The model under review builds one solid part; all positions refer to its coordinate system, in mm. A direction names the side the tool comes from. Coordinates: 2 decimals unless noted, no trailing zeros. Write each loop counter-clockwise with the first axis right and the second up, starting at its lowest first coordinate (ties: lowest second). Pieces come first, ordered by that corner, then holes. Notation, with made-up numbers: (-35, -29) - (-30, -29) arc R16 cw to (-30, -6) - close; hole circle Ø11 at (76, -34.75). An arc over 180 degrees is marked (long way). Put each result on its own line as item: value. Start each with the question number.
Item 1: Mouldability with a two-part tool opening along Y and no side actions: class faces 1 (the face through (-4.5, 0, 2)), 2 (the face through (0, -2.25, 2)), 3 (the face through (2, -1.75, 2)) as pulls with the +Y half, pulls with the -Y half, needs draft (parallel to the pull), parting line crosses it, or undercut.
Item 2: Consider section C-C on z = 4.3. State how many separate pieces and enclosed holes the cut face has, then the cut area to 3 significant figures.
Item 3: For pin 1 (1.8 mm diameter, centred on x = 2, y = -0.5, fed in from +Z), flat-tipped, find the tip position at first contact; note if it passes through.
Item 4: Consider section B-B on y = 1.6. Give the boundary of the cut face in (x, z), then the cut area to 3 significant figures.
Item 5: Machinability: for faces 4 (the face through (0, 0, -0.5)), 5 (the face through (-4, 0, 2)), which of the approach directions +Z, -Z, +X, -X, +Y, -Y give a long, thin tool a straight path to every point of the face, cutting with its end or side? Answer none if there is none.
Item 6: To check wall thickness, follow L1, parallel to X at y = -1.5, z = 3.6; L2, parallel to Y at x = -2.25, z = 3.5; L3, parallel to Y at x = 1.75, z = 4.5. State the ranges of each line that lie inside material, in increasing order. Write a range as [from, to].
Item 7: Consider section A-A on z = 1.6. Give the boundary of the cut face in (x, y).
```python
from build123d import *

# Parameters (mm, degrees)
SKETCH1_W             = 0.5
SKETCH1_H             = 4.5
EXTRUDE_THIN2_DEPTH   = 5
SKETCH1_W_2           = 9
SKETCH1_W_3           = 8
SKETCH1_H_2           = 3.5
EXTRUDE_THIN2_2_DEPTH = 5
SKETCH2_W             = 9
SKETCH2_H             = 4.5
BOSS_EXTRUDE1_DEPTH   = 0.5
SKETCH4_R             = 1.5
BOSS_EXTRUDE3_DEPTH   = 4.8
BOSS_EXTRUDE3_TAPER   = 4
FILLET1_R             = 1


with BuildPart() as part:
    # Sketch1 → Extrude-Thin2 (new body)
    with BuildSketch(Plane.XY):
        with Locations((0.25, 0)):
            Rectangle(SKETCH1_W, SKETCH1_H)
    extrude(amount=EXTRUDE_THIN2_DEPTH)



with BuildPart() as body_2:
    # Sketch1 → Extrude-Thin2 2 (new body)
    with BuildSketch(Plane.XY):
        Rectangle(SKETCH1_W_2, SKETCH1_H)
        Rectangle(SKETCH1_W_3, SKETCH1_H_2, mode=Mode.SUBTRACT)
    extrude(amount=EXTRUDE_THIN2_2_DEPTH)


with BuildPart() as part_1:
    add(part.part)

    add(body_2.part)  # Boss-Extrude1 merges body 2
    # Sketch2 → Boss-Extrude1 (add)
    with BuildSketch(Plane(origin=(0, 0, 0), x_dir=(-1, 0, 0), z_dir=(0, 0, -1))):
        Rectangle(SKETCH2_W, SKETCH2_H)
    extrude(amount=BOSS_EXTRUDE1_DEPTH)

    # Sketch4 → Boss-Extrude3 (add)
    with BuildSketch(Plane.XY):
        with Locations((2.25, 0)):
            Circle(SKETCH4_R)
        with Locations((-2, 0)):
            Circle(SKETCH4_R)
    extrude(amount=BOSS_EXTRUDE3_DEPTH, taper=BOSS_EXTRUDE3_TAPER)

    # Fillet1
    fillet1_edges = [part_1.edges().sort_by_distance(p)[0] for p in [
        (1.085648697, 0, 4.8),
        (-3.164351303, 0, 4.8),
    ]]
    fillet(fillet1_edges, radius=FILLET1_R)


solid = part_1.part
```
Report:
1. face 1: needs draft
1. face 2: pulls with the -Y half
1. face 3: undercut
2. separate pieces: 3
2. enclosed holes: 2
2. area: 21.8 mm²
3. pin 1: z = 4.8
4. outline: (-4.5, -0.5) - (4.5, -0.5) - (4.5, 5) - (4, 5) - (4, 0) - (0.5, 0) - (0.5, 5) - (0, 5) - (0, 0) - (-4, 0) - (-4, 5) - (-4.5, 5) - close
4. area: 12.0 mm²
5. face 4: -Z, +X, -X, +Y, -Y
5. face 5: +Z
6. L1: [-4.5, -4], [0, 0.5], [4, 4.5]
6. L2: [-2.25, -1.75], [-1.23, 1.23], [1.75, 2.25]
6. L3: [-2.25, -1.75], [-0.8, 0.8], [1.75, 2.25]
7. outline: (-4.5, -2.25) - (4.5, -2.25) - (4.5, 2.25) - (-4.5, 2.25) - close; circle Ø2.78 at (-2, 0); circle Ø2.78 at (2.25, 0); hole (-4, -1.75) - (0, -1.75) - (0, 1.75) - (-4, 1.75) - close; hole (0.5, -1.75) - (4, -1.75) - (4, 1.75) - (0.5, 1.75) - close
